```python
from build123d import *

# Parameters (mm, degrees)
F0_W     = 12.7
F0_H     = 6.35
F1_DEPTH = 0.79375
F2_W     = 4.7625
F2_H     = 1.27
F3_DEPTH = 25.4
F4_R     = 0.381
F2_W_2   = 12.7
F2_H_2   = 3.175
F5_DEPTH = 1.5875
F6_R     = 1.5748
F6_R_2   = 1.27
F7_DEPTH = 0.889
F9_R     = 0.254


# Not quite as in the source:
# - a fillet or chamfer that OpenCascade refuses, or shapes differently, is made with other operations: its cross-section is extruded or revolved along the edge and cut away or added


with BuildPart() as f1:
    # F0 (on Front) → F1 (new body)
    with BuildSketch(Plane.XZ):
        Rectangle(F0_W, F0_H)
    extrude(amount=F1_DEPTH)

    # F2 (on face) → F3 (cut)
    with BuildSketch(Plane.XZ.offset(0.79375)):
        with Locations((-3.96875, -2.54)):
            Rectangle(F2_W, F2_H)
        with Locations((3.96875, -2.54)):
            Rectangle(F2_W, F2_H)
    extrude(amount=-F3_DEPTH, mode=Mode.SUBTRACT)

    # F4
    f4_edges = [f1.edges().sort_by_distance(p)[0] for p in [
        (-1.5875, -0.396875, -3.175),
        (1.5875, -0.396875, -3.175),
        (-6.35, -0.396875, -1.905),
        (6.35, -0.396875, -1.905),
        (1.5875, -0.396875, -1.905),
        (-1.5875, -0.396875, -1.905),
    ]]
    fillet(f4_edges, radius=F4_R)

    # F2 (on face) → F5 (join)
    with BuildSketch(Plane.XZ.offset(0.79375)):
        with Locations((0, 1.5875)):
            Rectangle(F2_W_2, F2_H_2)
    extrude(amount=F5_DEPTH)

    # F6 (on face) → F7 (cut)
    with BuildSketch(Plane.XZ.offset(2.38125)):
        with Locations((-3.175, 1.5875)):
            Circle(F6_R)
        with Locations((-3.175, 1.5875)):
            Circle(F6_R_2, mode=Mode.SUBTRACT)
        with Locations((3.175, 1.5875)):
            Circle(F6_R)
        with Locations((3.175, 1.5875)):
            Circle(F6_R_2, mode=Mode.SUBTRACT)
    extrude(amount=-F7_DEPTH, mode=Mode.SUBTRACT)

    # F8: chamfer of 0.381 on 2 edges, made by hand

    # F8_s1 → F8_t2 (revolve)
    with BuildSketch(Plane.XY.offset(1.5875)):
        Polygon((-1.6002, -1.87325), (-1.9812, -1.49225), (-1.6002, -1.49225), align=None)
    revolve(axis=Axis((-3.175, -1.49225, 1.5875), (0, -1, 0)))

    # F8_s3 → F8_t4 (revolve)
    with BuildSketch(Plane.XY.offset(1.5875)):
        Polygon((4.7498, -1.87325), (4.3688, -1.49225), (4.7498, -1.49225), align=None)
    revolve(axis=Axis((3.175, -1.49225, 1.5875), (0, -1, 0)))

    # F9
    f9_edges = [f1.edges().sort_by_distance(p)[0] for p in [
        (-4.445, -2.38125, 1.5875),
        (1.905, -2.38125, 1.5875),
    ]]
    fillet(f9_edges, radius=F9_R)


solid = f1.part
```
The model under review builds one solid part; all positions refer to its coordinate system, in mm. A direction names the side the tool comes from. Give positions to 0.01 mm unless a question says otherwise; leave off trailing zeros. Loops run counter-clockwise (first coordinate to the right, second up) from the corner with the lowest first, then second, coordinate; pieces in that order, holes last. Notation, with made-up numbers: (11, 34.25) - (51, 34.25) arc R20 ccw to (51, 61.25) - close; hole circle Ø8 at (10, -31). An arc over 180 degrees is marked (long way). Answer as a JSON object with one key per item and string values.
Q1. For faces 1 (the flat face through (3, -2.381, 2)), 2 (the flat face through (0, -2, 0)), 3 (the cylindrical face through (-1.72, -2.13, 0.98)), list the 3-axis set-ups (+Z, -Z, +X, -X, +Y, -Y) from which the entire face can be reached by the end or side of a thin tool; tool diameter is ignored.
Worked out:
{"face 1": "+Z, -Z, +X, -X, -Y", "face 2": "-Z, +X, -X, -Y", "face 3": "-Y"}
Q2. Add section D-D on z = -1. State the section outline as (x, y) points.
Worked out:
{"outline": "(-6.35, -0.79) - (6.35, -0.79) - (6.35, 0) - (-6.35, 0) - close"}
Q3. Add section B-B on x = 0. State the section outline as (y, z) points (3 decimals), plus the area to 3 significant figures.
Worked out:
{"outline": "(-2.381, 0) - (-0.794, 0) - (-0.794, -3.175) - (0, -3.175) - (0, 3.175) - (-2.381, 3.175) - close", "area": "10.1 mm^2"}
Q4. Mouldability with a two-part tool opening along X and no side actions: class faces 4 (the flat face through (6.35, -1, 1)), 5 (the cylindrical face through (4.63, -2.13, 0.98)), 6 (the flat face through (0, -1, 3.175)) as +X half, -X half, draft (parallel to the pull), parting line (faces both ways), or undercut.
Worked out:
{"face 4": "+X half", "face 5": "undercut", "face 6": "draft"}
Q5. To check wall thickness, follow line 1 along X through (y, z) = (-2, 3); line 2 along Z through (x, y) = (-2.25, -2.15) (3 decimals); line 3 along Y through (x, z) = (2, -1.75). State the ranges of each line that lie inside material, in increasing order.
Worked out:
{"line 1": "x = -6.35 to -3.87, -2.48 to 2.48, 3.87 to 6.35", "line 2": "z = 0 to 0.313, 0.719 to 2.456, 2.862 to 3.175", "line 3": "y = -0.79 to 0"}
Q6. Insertion check: pin 1 (0.8 mm diameter, centred on x = 2.5, y = -1.5, fed in from -Z); pin 2 (1.6 mm diameter, centred on x = -2, z = -1, fed in from -Y); pin 3 (0.6 mm diameter, centred on y = -0.5, z = -2.5, fed in from -X); pin 4 (1.9 mm diameter, centred on x = -3.18, z = 1.59, fed in from +Y). Each pin has a flat end and moves straight along its axis. Give the tip position at first contact, or say it passes through.
Worked out:
{"pin 1": "stops at z = 0", "pin 2": "stops at y = -0.79", "pin 3": "stops at x = -1.6", "pin 4": "stops at y = 0"}
Q7. Add section A-A on y = -1.7. Count the separate pieces of the cut face and the enclosed holes in it, plus the area to 3 significant figures.
Worked out:
{"separate pieces": "3", "enclosed holes": "2", "area": "38.1 mm^2"}
